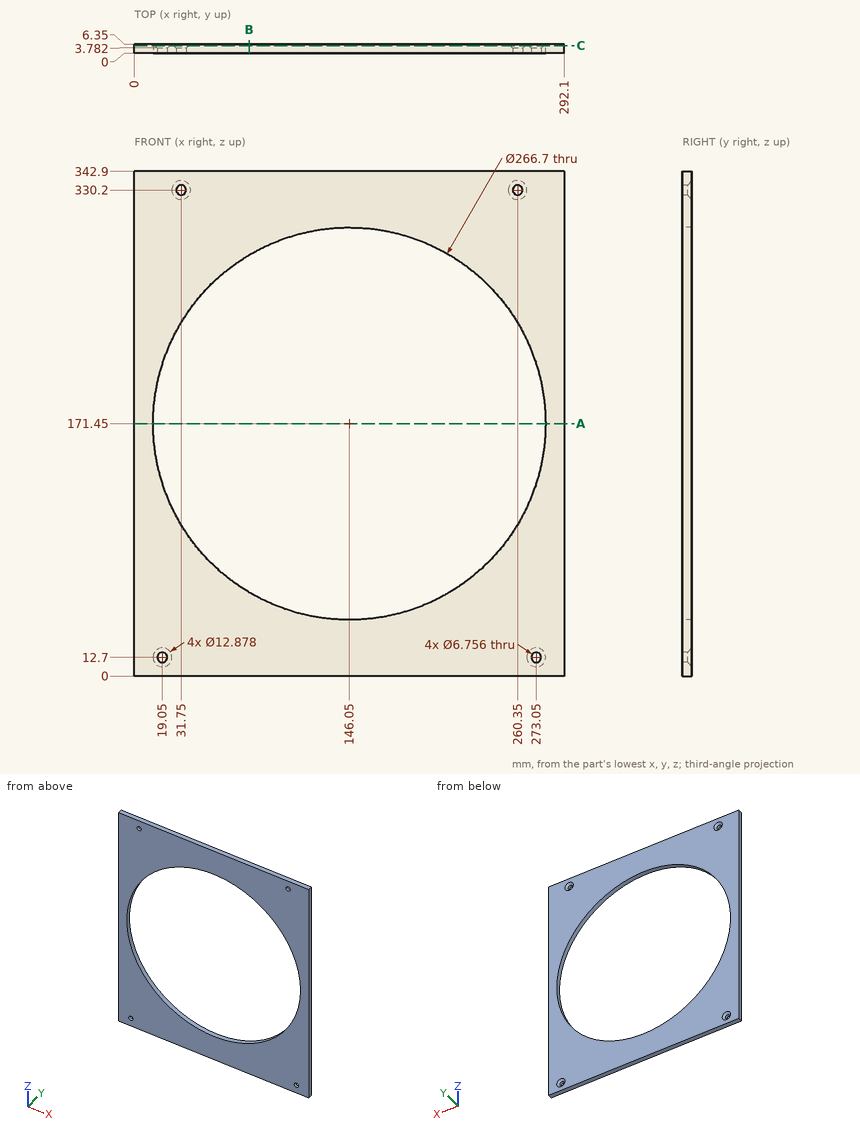
Study the drawing (mm; zero at the part's minimum x, y, z) and answer. Give positions to 0.01 mm unless a question says otherwise; leave off trailing zeros. Write each loop counter-clockwise with the first axis right and the second up, starting at its lowest first coordinate (ties: lowest second). Pieces come first, ordered by that corner, then holes.
Item 1: Section A-A, the plane z = 171.45 is taken. Write down the section's boundary in (x, y).
Item 2: A flat-ended cylindrical pin translates along its axis: P1, Ø5.5, axis at x = 31.75, z = 330.2, coming from the -Y side. Find the tip coordinate at first contact, or state that the pin passes through.
Item 3: Section B-B, the plane x = 78 is taken. Write down the section's boundary in (y, z).
Item 4: Section C-C, the plane y = 5.25 is taken. Write down the section's boundary in (x, z).
Item 5: Find the intervals of material crossed by line 1 along X through (y, z) = (3, 12.7); line 2 along X through (y, z) = (2.75, 198); line 3 along Z through (x, y) = (149, 1.75), in increasing order.
Completed:
1. outline: (0, 0) - (12.7, 0) - (12.7, 6.35) - (0, 6.35) - close; (279.4, 0) - (292.1, 0) - (292.1, 6.35) - (279.4, 6.35) - close
2. P1: passes through
3. outline: (0, 0) - (6.35, 0) - (6.35, 56.77) - (0, 56.77) - close; (0, 286.13) - (6.35, 286.13) - (6.35, 342.9) - (0, 342.9) - close
4. outline: (0, 0) - (292.1, 0) - (292.1, 342.9) - (0, 342.9) - close; hole circle Ø266.7 at (146.05, 171.45); hole circle Ø10.26 at (19.05, 12.7); hole circle Ø10.26 at (31.75, 330.2); hole circle Ø10.26 at (260.35, 330.2); hole circle Ø10.26 at (273.05, 12.7)
5. line 1: x = 0 to 15.67, 22.43 to 269.67, 276.43 to 292.1
5. line 2: x = 0 to 15.37, 276.73 to 292.1
5. line 3: z = 0 to 38.13, 304.77 to 342.9
